from build123d import *

# Parameters (mm, degrees)
SKETCH1_W           = 26.5
SKETCH1_H           = 43.65
BOSS_EXTRUDE1_DEPTH = 1.5
FILLET1_R           = 3.15
SKETCH2_R           = 1.575
CUT_EXTRUDE1_DEPTH  = 1.5
SKETCH3_W           = 15
SKETCH3_H           = 18.8
BOSS_EXTRUDE2_DEPTH = 15.8


with BuildPart() as part:
    # Sketch1 → Boss-Extrude1 (new body)
    with BuildSketch(Plane(origin=(0, 0, 0), x_dir=(1, 0, 0), z_dir=(0, 1, 0))):
        Rectangle(SKETCH1_W, SKETCH1_H)
    extrude(amount=BOSS_EXTRUDE1_DEPTH)

    # Fillet1
    fillet1_edges = [part.edges().sort_by_distance(p)[0] for p in [
        (-13.25, 0.75, -21.825),
        (13.25, 0.75, -21.825),
        (13.25, 0.75, 21.825),
        (-13.25, 0.75, 21.825),
    ]]
    fillet(fillet1_edges, radius=FILLET1_R)

    # Sketch2 → Cut-Extrude1 (cut)
    with BuildSketch(Plane(origin=(0, 1.5, 0), x_dir=(1, 0, 0), z_dir=(0, 1, 0))):
        with Locations(Location((-10.725, 19.05, 0), (0, 0, 270))):
            Circle(SKETCH2_R)
        with Locations(Location((10.725, 19.05, 0), (0, 0, 270))):
            Circle(SKETCH2_R)
        with Locations(Location((10.725, -19.05, 0), (0, 0, 270))):
            Circle(SKETCH2_R)
        with Locations(Location((-10.725, -19.05, 0), (0, 0, 270))):
            Circle(SKETCH2_R)
    extrude(amount=-CUT_EXTRUDE1_DEPTH, mode=Mode.SUBTRACT)

    # Sketch3 → Boss-Extrude2 (add)
    with BuildSketch(Plane(origin=(0, 1.5, 0), x_dir=(1, 0, 0), z_dir=(0, 1, 0))):
        with Locations((0, -2.375)):
            Rectangle(SKETCH3_W, SKETCH3_H)
    extrude(amount=BOSS_EXTRUDE2_DEPTH)


solid = part.part
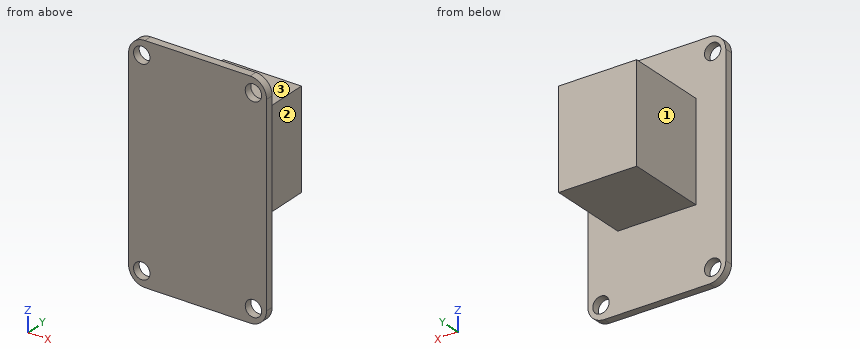
Part model, mm, in its own coordinate system. Face numbers are marked on the shaded views. A direction names the side the tool comes from. Give positions to 0.01 mm unless a question says otherwise; leave off trailing zeros. Write each loop counter-clockwise with the first axis right and the second up, starting at its lowest first coordinate (ties: lowest second). Pieces come first, ordered by that corner, then holes.
1) Cut at B-B on x = 8.25. Write the cut outline in (y, z) (3 decimals), then the cut area to 3 significant figures.
Resolved:
outline: (0, -21.825) - (1.5, -21.825) - (1.5, 21.825) - (0, 21.825) - close
area: 65.5 mm2
2) Which spindle directions (+Z, -Z, +X, -X, +Y, -Y) get a long thin tool onto all of the face, cutting with end or side? Do the marked faces 1, 2 and 3. Say none if no direction does.
Resolved:
face 1: +Z, -Z, -X, +Y
face 2: +Z, -Z, +X, +Y
face 3: +Z, +X, -X, +Y
3) Pin check, flat tips, straight feed: pin 1 (2 mm diameter, centred on x = -2, z = -11.5, fed in from +Y); pin 2 (7.5 mm diameter, centred on x = -1, y = 5.5, fed in from +Z) (3 decimals); pin 3 (3 mm diameter, centred on x = -10.725, z = -19.05, fed in from +Y); pin 4 (8 mm diameter, centred on y = 10.5, z = 5.5, fed in from -X). Stop position of each tip, or through.
Resolved:
pin 1: stops at y = 1.5
pin 2: stops at z = 11.775
pin 3: passes through
pin 4: stops at x = -7.5
4) Cut at C-C on y = 10.5. Write the cut outline in (x, z) (3 decimals).
Resolved:
outline: (-7.5, -7.025) - (7.5, -7.025) - (7.5, 11.775) - (-7.5, 11.775) - close
5) Cut at A-A on z = 3.5. Write the cut outline in (x, y), then the cut area to 3 significant figures.
Resolved:
outline: (-13.25, 0) - (13.25, 0) - (13.25, 1.5) - (7.5, 1.5) - (7.5, 17.3) - (-7.5, 17.3) - (-7.5, 1.5) - (-13.25, 1.5) - close
area: 277 mm2
6) Probe L1, parallel to Y at x = -7.5, z = -14; L2, parallel to Z at x = 7, y = 6 (3 decimals); L3, parallel to X at y = 0.8, z = -19.05. List the from-to ranges inside material, lowest first.
Resolved:
L1: y = 0 to 1.5
L2: z = -7.025 to 11.775
L3: x = -13.23 to -12.3, -9.15 to 9.15, 12.3 to 13.23
